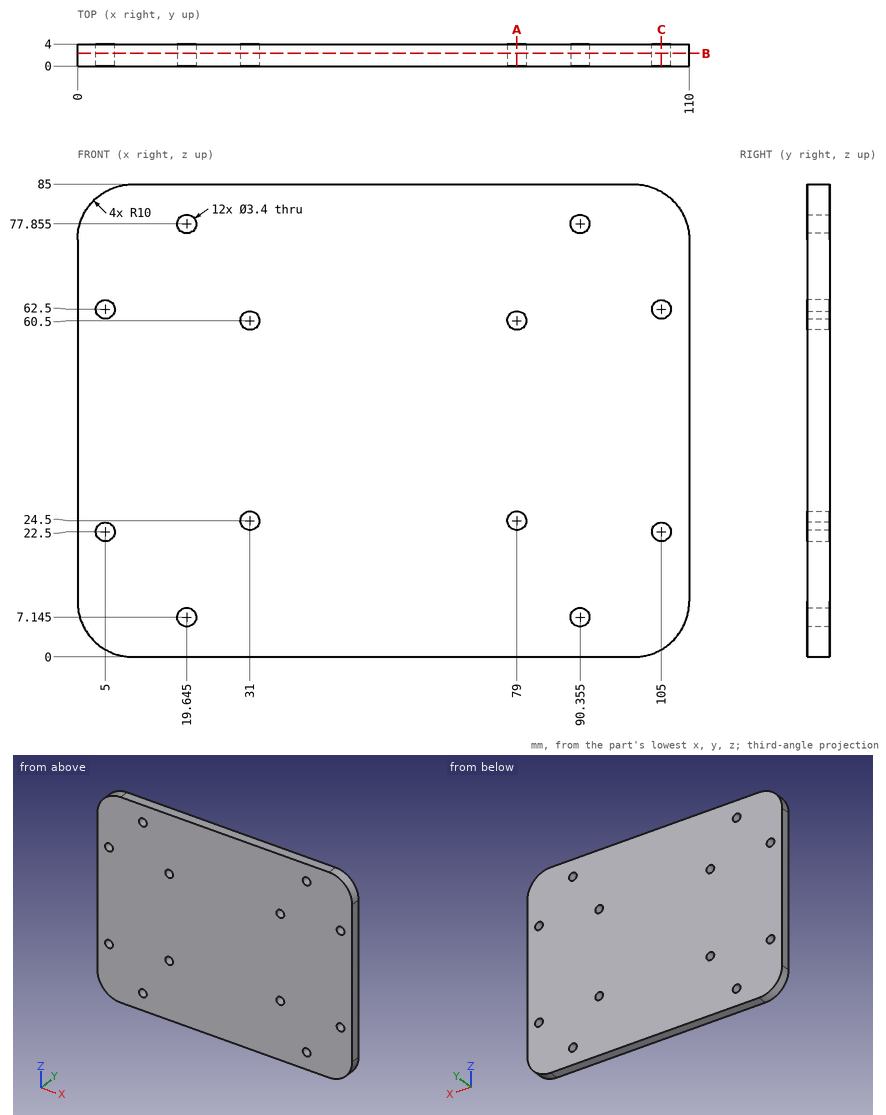
Source: three-view drawing plus pictorial views. Frame: mm from the lowest corner of the part. Coordinates: 2 decimals unless noted, no trailing zeros. Loops run counter-clockwise (first coordinate to the right, second up) from the corner with the lowest first, then second, coordinate; pieces in that order, holes last. Notation, with made-up numbers: (26.25, -12.5) - (82.25, -12.5) arc R15 cw to (82.25, 14.5) - close; hole circle Ø3 at (62, 78). An arc over 180 degrees is marked (long way). One line per item, written item: value. Start each with the question number.
1. Ray query, L1, parallel to Z at x = 79, y = 3; L2, parallel to Z at x = 90.5, y = 2.65; L3, parallel to X at y = 1.9, z = 62.5. Return the intervals inside material, ascending.
2. Section A-A (x = 79). Return the cut outline in (y, z).
3. Section C-C (x = 105). Return the cut outline in (y, z), and give its area (3 significant figures).
4. Contact query for a flat-ended pin moving along its axis: P1, Ø3, axis at x = 31, z = 24.5, coming from the -Y side (3 decimals). Output: stop coordinate, or through.
5. Section B-B (y = 2.3). State how many separate pieces and enclosed holes the cut face has, and give its area (3 significant figures).
Verdict:
1. L1: z = 0 to 22.8, 26.2 to 58.8, 62.2 to 85
1. L2: z = 0 to 5.45, 8.84 to 76.16, 79.55 to 85
1. L3: x = 0 to 3.3, 6.7 to 103.3, 106.7 to 110
2. outline: (0, 0) - (4, 0) - (4, 22.8) - (0, 22.8) - close; (0, 26.2) - (4, 26.2) - (4, 58.8) - (0, 58.8) - close; (0, 62.2) - (4, 62.2) - (4, 85) - (0, 85) - close
3. outline: (0, 1.34) - (4, 1.34) - (4, 20.8) - (0, 20.8) - close; (0, 24.2) - (4, 24.2) - (4, 60.8) - (0, 60.8) - close; (0, 64.2) - (4, 64.2) - (4, 83.66) - (0, 83.66) - close
3. area: 302 mm2
4. P1: passes through
5. separate pieces: 1
5. enclosed holes: 12
5. area: 9,160 mm2
